For this review, use the dimensioned drawing (mm, ordinates from the lowest corner) and the shaded views. A direction names the side the tool comes from. Coordinates: 2 decimals unless noted, no trailing zeros. Loops run counter-clockwise (first coordinate to the right, second up) from the corner with the lowest first, then second, coordinate; pieces in that order, holes last. Notation, with made-up numbers: (49, -9.5) -> (62, -9.5) arc R25 ccw to (62, 5.5) -> close; hole circle Ø4 at (59.5, 57.25). An arc over 180 degrees is marked (long way). Use one line per item in the form item = value. Start each with the question number.
1. Consider section D-D (z = 33.5). State the section outline as (x, y) points.
2. Consider section A-A (y = 27). State the section outline as (x, z) points, then the cut area to 3 significant figures.
3. Machinability: for the marked faces 5 and 6, which of the approach directions +Z, -Z, +X, -X, +Y, -Y give a long, thin tool a straight path to every point of the face, cutting with its end or side? Answer none if there is none.
4. Wall thickness on line 1 (X direction, y = 11.5, z = 9); line 2 (Y direction, x = 36, z = 5); line 3 (Z direction, x = 37, y = 27): over which ranges is each line inside the solid? List them lowest first. Write a range as from..to.
5. The part is to be moulded in two halves that separate along X. For the marked faces 1, 2, 3 and 4, say which applies: released by +X, released by -X, zero draft, split by the parting line, or undercut.
6. Consider section C-C (x = 14). State the section outline as (y, z) points, then the cut area to 3 significant figures.
7. For pin 1 (2 mm diameter, centred on x = 14.5, y = 10, fed in from +Z); pin 2 (1 mm diameter, centred on x = 12, y = 17.5, fed in from +Z); pin 3 (5 mm diameter, centred on x = 15, y = 11.5, fed in from -Z), all flat-tipped, find the tip position at first contact; note any pin that passes through.
8. Consider section B-B (x = 28.5). State the section outline as (y, z) points.
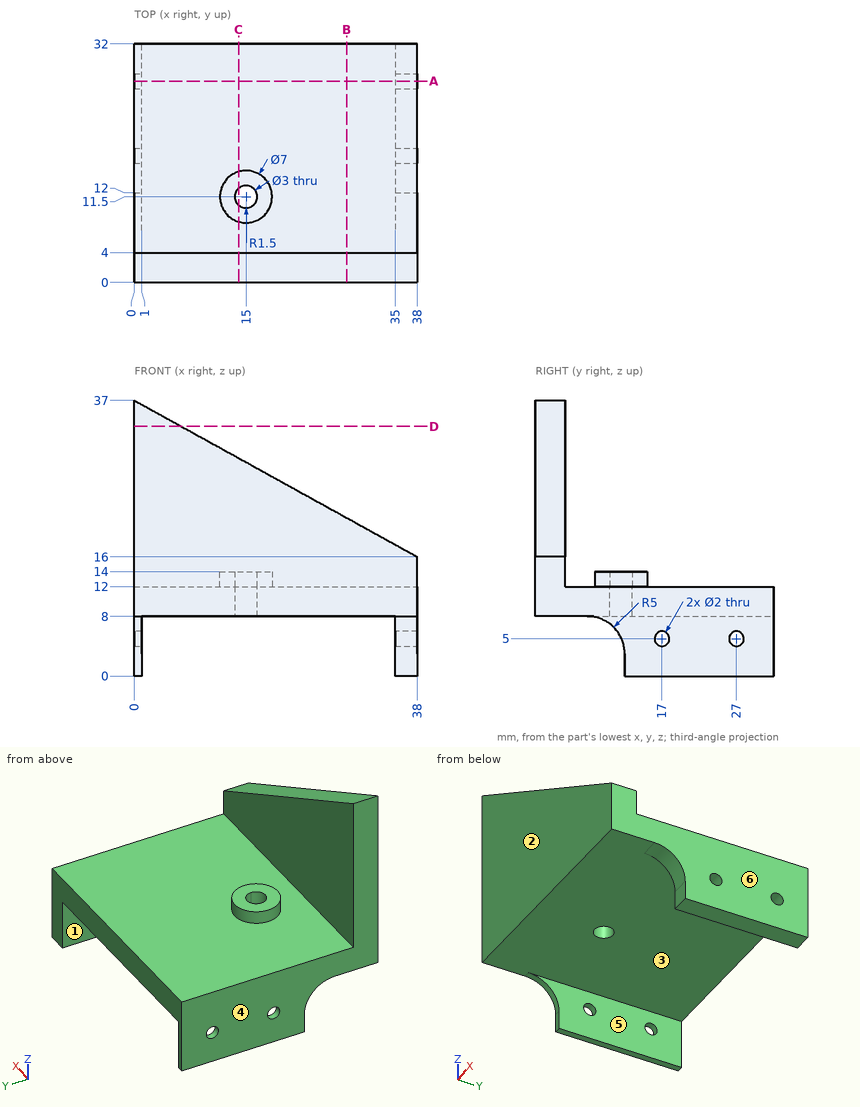
Geometry check:
q1.outline = (0, 0) -> (6.33, 0) -> (6.33, 4) -> (0, 4) -> close
q2.outline = (0, 0) -> (1, 0) -> (1, 4) -> (0, 4) -> close; (0, 6) -> (1, 6) -> (1, 8) -> (35, 8) -> (35, 6) -> (38, 6) -> (38, 12) -> (0, 12) -> close; (35, 0) -> (38, 0) -> (38, 4) -> (35, 4) -> close
q2.area = 176 mm²
q3.face_5 = -Z, +Y, -Y
q3.face_6 = +Z, -Z, +X, +Y, -Y
q4.line_1 = 0..13.5, 16.5..38
q4.line_2 = 11.58..16, 18..26, 28..32
q4.line_3 = 0..4, 6..12
q5.face_1 = undercut
q5.face_2 = zero draft
q5.face_3 = undercut
q5.face_4 = released by -X
q6.outline = (0, 8) -> (10.38, 8) -> (10.38, 14) -> (8.15, 14) -> (8.15, 12) -> (4, 12) -> (4, 29.26) -> (0, 29.26) -> close; (12.62, 8) -> (32, 8) -> (32, 12) -> (14.85, 12) -> (14.85, 14) -> (12.62, 14) -> close
q6.area = 197 mm²
q7.pin_1 = 14
q7.pin_2 = 12
q7.pin_3 = 8
q8.outline = (0, 8) -> (32, 8) -> (32, 12) -> (4, 12) -> (4, 21.25) -> (0, 21.25) -> close
